Autodesk Inventor part; units mm, degrees
ref_plane "YZ Plane" through (0, 0, 0) normal (1, 0, 0) x (0, 1, 0)
ref_plane "XZ Plane" through (0, 0, 0) normal (0, 1, 0) x (-1, 0, 0)
ref_plane "XY Plane" through (0, 0, 0) normal (0, 0, 1) x (1, 0, 0)
sketch "Sketch1" plane through (0, 0, 0) normal (1, 0, 0) x (0, 1, 0)
  line L0 (0, 0) -> (0, 25.4)
  line L1 (0, 25.4) -> (203.2, 25.4)
  line L2 (203.2, 25.4) -> (203.2, 0)
  line L3 (203.2, 0) -> (201.6125, 0)
  line L4 (201.6125, 0) -> (201.6125, 23.8125)
  line L5 (201.6125, 23.8125) -> (1.5875, 23.8125)
  line L6 (1.5875, 23.8125) -> (1.5875, 0)
  line L7 (1.5875, 0) -> (0, 0)
  dimension "d0" = 25.4
  dimension "d1" = 203.2
  dimension "d2" = 1.5875
  dimension "d3" = 1.5875
  dimension "d4" = 1.5875
  dimension "d5" = 25.4
extrude "Extrusion1" add sketch "Sketch1" along normal blind 25.4
sketch "Sketch2" plane through (0, 203.2, 25.4) normal (0, 1, 0) x (1, 0, 0)
  line L0 (25.4, 25.4) -> (25.4, 0)
  line L1 (0, 25.4) -> (25.4, 25.4)
  point P0 (12.7, 12.7)
  dimension "d8" = 12.7
  dimension "d9" = 12.7
hole "Hole1" at (12.7, 203.2, 12.7) direction (0, -1, 0) diameter 6.35 end through all
sketch "Sketch3" plane through (0, 0, 25.4) normal (0, 0, 1) x (1, 0, 0)
  line L0 (0, 0) -> (0, 203.2)
  line L1 (0, 0) -> (25.4, 0)
  line L2 (25.4, 203.2) -> (25.4, 0)
  line L3 (0, 101.6) -> (25.4, 101.6)
  point P0 (12.7, 127)
  point P1 (12.7, 76.2)
  dimension "d17" = 12.7
  dimension "d18" = 12.7
  dimension "d28" = 101.6
  dimension "d29" = 50.8
  dimension "d30" = 25.4
hole "Hole2" at (12.7, 127, 25.4) at (12.7, 76.2, 25.4) direction (0, 0, -1) diameter 6.35 end through all
properties part number "SupportBAr" material "Aluminum 6061"
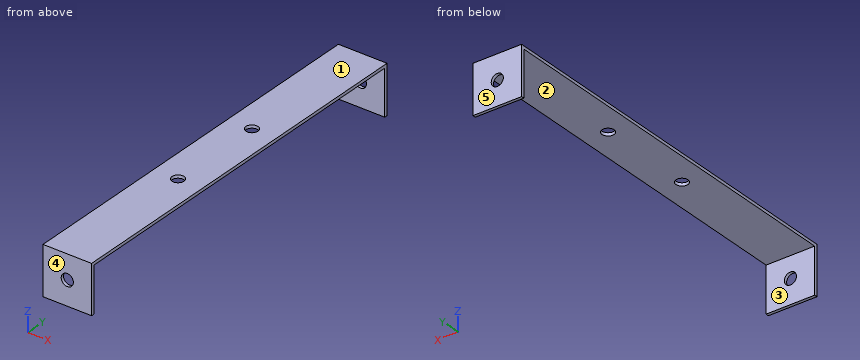
Input: part model. Units: mm. Frame: model coordinates. Face numbers are marked on the shaded views. A direction names the side the tool comes from. Round coordinates to 2 decimals unless told otherwise and drop trailing zeros. Loops run counter-clockwise (first coordinate to the right, second up) from the corner with the lowest first, then second, coordinate; pieces in that order, holes last.
1) Material intervals for line 1 (Y direction, x = 12.7, z = 24.55) (3 decimals); line 2 (Y direction, x = 1.75, z = 22.25); line 3 (X direction, y = 1.15, z = 12.7) (3 decimals), sorted ascending.
Ans:
line 1: y = 0 to 73.025, 79.375 to 123.825, 130.175 to 203.2
line 2: y = 0 to 1.59, 201.61 to 203.2
line 3: x = 0 to 9.525, 15.875 to 25.4
2) Section query A-A on x = 12.7. Return the cut outline in (y, z) (1 decimal).
Ans:
outline: (0, 0) - (1.6, 0) - (1.6, 9.5) - (0, 9.5) - close; (0, 15.9) - (1.6, 15.9) - (1.6, 23.8) - (73, 23.8) - (73, 25.4) - (0, 25.4) - close; (79.4, 23.8) - (123.8, 23.8) - (123.8, 25.4) - (79.4, 25.4) - close; (130.2, 23.8) - (201.6, 23.8) - (201.6, 15.9) - (203.2, 15.9) - (203.2, 25.4) - (130.2, 25.4) - close; (201.6, 0) - (203.2, 0) - (203.2, 9.5) - (201.6, 9.5) - close
3) Pin query (flat end, axial travel): pin 1 (10 mm diameter, centred on x = 12.7, y = 76.2, fed in from -Z); pin 2 (6 mm diameter, centred on x = 9.5, z = 17, fed in from -Y). Return the tip coordinate at first contact, or that it passes through.
Ans:
pin 1: stops at z = 23.81
pin 2: stops at y = 0
4) Pull-direction query (Y, two-part tool) for the marked faces 3, 4 and 5; classes: released by +Y, released by -Y, zero draft, split by the parting line, or undercut.
Ans:
face 3: undercut
face 4: released by -Y
face 5: released by +Y
5) Section query C-C on y = 76.2. Return the cut outline in (x, z) (1 decimal), plus the area to 3 significant figures.
Ans:
outline: (0, 23.8) - (9.5, 23.8) - (9.5, 25.4) - (0, 25.4) - close; (15.9, 23.8) - (25.4, 23.8) - (25.4, 25.4) - (15.9, 25.4) - close
area: 30.2 mm2
6) Set-up query: the marked faces 1 and 2. Return all of +Z, -Z, +X, -X, +Y, -Y with unobstructed straight access to the full face (end or side cutting, diameter ignored); none if empty.
Ans:
face 1: +Z, +X, -X, +Y, -Y
face 2: -Z, +X, -X
7) Section query D-D on z = 12.25. Return the cut outline in (x, y).
Ans:
outline: (0, 0) - (9.56, 0) - (9.56, 1.59) - (0, 1.59) - close; (0, 201.61) - (9.56, 201.61) - (9.56, 203.2) - (0, 203.2) - close; (15.84, 0) - (25.4, 0) - (25.4, 1.59) - (15.84, 1.59) - close; (15.84, 201.61) - (25.4, 201.61) - (25.4, 203.2) - (15.84, 203.2) - close
8) Section query B-B on z = 21.25. Return the cut outline in (x, y).
Ans:
outline: (0, 0) - (25.4, 0) - (25.4, 1.59) - (0, 1.59) - close; (0, 201.61) - (25.4, 201.61) - (25.4, 203.2) - (0, 203.2) - close
